Build history of the part. All positions in model axes, mm. A direction names the side the tool comes from. Round coordinates to 2 decimals unless told otherwise and drop trailing zeros. Order: outer loops, then holes, each group sorted by start corner. A loop starts at its lowest first (then second) coordinate and runs counter-clockwise, first axis right, second up. Notation, with made-up numbers: (17, 36) -> (26, 36) arc R19 ccw to (26, 53) -> close; hole circle Ø4 at (-27, 66). An arc over 180 degrees is marked (long way). Answer as CSV lines item,"result". Start each with the question number.
Autodesk Inventor part; units mm, degrees
ref_plane "YZ Plane" through (0, 0, 0) normal (1, 0, 0) x (0, 1, 0)
ref_plane "XZ Plane" through (0, 0, 0) normal (0, 1, 0) x (-1, 0, 0)
ref_plane "XY Plane" through (0, 0, 0) normal (0, 0, 1) x (1, 0, 0)
sketch "Náčrt1" plane through (0, 0, 0) normal (0, 1, 0) x (-1, 0, 0)
  line L0 (0, -68.6) -> (0, 68.6)
  line L1 (-123.9, 0) -> (123.9, 0)
  line L2 (88.5, -49) -> (-88.5, -49)
  line L3 (-88.5, -49) -> (-88.5, 49)
  line L4 (-88.5, 49) -> (88.5, 49)
  line L5 (88.5, 49) -> (88.5, -49)
  point P0 (0, 0)
  dimension "d0" = 177
  dimension "d1" = 98
extrude "Vysunutí1" add sketch "Náčrt1" along normal blind 3
sketch "Náčrt2" plane through (0, 3, 0) normal (0, 1, 0) x (1, 0, 0)
  line L0 (0, 68.6) -> (0, -68.6)
  line L1 (123.9, 0) -> (-123.9, 0)
  point P0 (0, 0)
  point P1 (-83.55, 44.05)
  point P2 (-83.55, -44.05)
  point P3 (83.55, -44.05)
  point P4 (83.55, 44.05)
  dimension "d4" = 88.1
  dimension "d5" = 167.1
  dimension "d6" = 88.1
  dimension "d7" = 167.1
hole "Díra1" at (-83.55, 3, -44.05) at (-83.55, 3, 44.05) at (83.55, 3, 44.05) at (83.55, 3, -44.05) direction (0, -1, 0) diameter 3.4 end through all
fillet "Zaoblení1" radius 3 4 edges at (88.5, 1.5, 49) (88.5, 1.5, -49) (-88.5, 1.5, 49) (-88.5, 1.5, -49)
sketch "Náčrt3" plane through (0, 3, 0) normal (0, 1, 0) x (1, 0, 0)
  line L0 (123.9, 0) -> (-123.9, 0)
  line L1 (-88.5, 46) -> (-88.5, -46)
  point P0 (0, 0)
  point P1 (-38.5, 0)
  dimension "d21" = 50
hole "Díra2" at (-38.5, 3, 0) direction (0, -1, 0) diameter 60.1 end through all
sketch "Náčrt4" plane through (0, 0, 0) normal (0, -1, 0) x (1, 0, 0)
  line L0 (0, 68.6) -> (0, -68.6)
  line L1 (-123.9, 0) -> (123.9, 0)
  point P0 (0, 0)
  point P1 (40, -15)
  dimension "d29" = 40
  dimension "d38" = 15
hole "Díra3" at (40, 0, -15) direction (0, 1, 0) diameter 47.3 end through all counterbore diameter 50.3 counterbore depth 1
sketch "Náčrt5" plane through (0, 3, 0) normal (0, 1, 0) x (1, 0, 0)
  line L0 (30.3, -22.5) -> (48.5, -22.5)
  line L1 (48.5, -22.5) -> (48.5, -34)
  line L2 (48.5, -34) -> (30.3, -34)
  line L3 (30.3, -34) -> (30.3, -22.5)
  line L4 (-85.5, -49) -> (85.5, -49)
  line L5 (88.5, -46) -> (88.5, 46)
  point P0 (0, 0)
  dimension "d39" = 18.2
  dimension "d40" = 11.5
  dimension "d41" = 15
  dimension "d43" = 40
extrude "Vysunutí2" cut sketch "Náčrt5" against normal up to surface (3 mm away)
sketch "Náčrt6" plane through (0, 3, 0) normal (0, 1, 0) x (1, 0, 0)
  line L0 (123.9, 0) -> (-123.9, 0)
  line L1 (0, 68.6) -> (0, -68.6)
  circle A0 centre (-38.5, 0) radius 30.05
  point P0 (0, 0)
  point P1 (-67.5, -29)
  point P2 (-9.5, 29)
  dimension "d46" = 29
  dimension "d49" = 29
  dimension "d57" = 29
  dimension "d58" = 29
hole "Díra4" at (-67.5, 3, 29) at (-9.5, 3, -29) direction (0, -1, 0) diameter 3.9 end through all
chamfer "Zkosení1" distance 1.5 angle 45 6 edges at (83.55, 3, -45.75) (-83.55, 3, -45.75) (83.55, 3, 42.35) (-83.55, 3, 42.35) (-9.5, 3, -30.95) (-67.5, 3, 27.05)
properties part number "4.L - GM - 01.02" material "LCP plast"
Q1. Which spindle directions (+Z, -Z, +X, -X, +Y, -Y) get a long thin tool onto all of the face, cutting with end or side? Do faces 1 (the face through (59, 1, -30)), 2 (the face through (32.9, 2.01, -37.56)). Say none if no direction does.
Q2. Slice it at C-C, the plane x = -38.5. Write the cut outline in (y, z), plus the area to 3 significant figures.
Q3. Slice it at A-A, the plane x = 40. Write the cut outline in (y, z).
Q4. Slice it at B-B, the plane z = -44.05. Write the cut outline in (x, y).
Q5. Two-plate mould, pull along X, no slides. Class faces 3 (the face through (-8.75, 0.74, -27.2)), 4 (the face through (1, 0, 1)): +X half, -X half, draft (parallel to the pull), parting line (faces both ways), or undercut.
Q6. Flat gauge pins, fed straight in: pin 1 Ø2.5 at (x, z) = (83.55, 44.05) entering from +Y; pin 2 Ø1 at (x, z) = (-69, -17.5) entering from -Y. Where does each tip first touch, or does it go through?
Q7. Probe L1, parallel to X at y = 0.95, z = -44.05; L2, parallel to Z at x = -83.55, y = 1.25; L3, parallel to Z at x = 40, y = 1.7. List the from-to ranges inside material, lowest first.
Q8. Slice it at D-D, the plane z = 12. Write the cut outline in (x, y).
Solutions:
1,face 1,"-Y"
1,face 2,"+Y, -Y"
2,outline,"(0, -49) -> (3, -49) -> (3, -30.05) -> (0, -30.05) -> close; (0, 30.05) -> (3, 30.05) -> (3, 49) -> (0, 49) -> close"
2,area,"114 mm2"
3,outline,"(0, -49) -> (3, -49) -> (3, -38.65) -> (1, -38.65) -> (1, -40.15) -> (0, -40.15) -> close; (0, 10.15) -> (1, 10.15) -> (1, 8.65) -> (3, 8.65) -> (3, 22.5) -> (0, 22.5) -> close; (0, 34) -> (3, 34) -> (3, 49) -> (0, 49) -> close"
4,outline,"(-88.5, 0) -> (-85.25, 0) -> (-85.25, 1.5) -> (-86.75, 3) -> (-88.5, 3) -> close; (-81.85, 0) -> (81.85, 0) -> (81.85, 1.5) -> (80.35, 3) -> (-80.35, 3) -> (-81.85, 1.5) -> close; (85.25, 0) -> (88.5, 0) -> (88.5, 3) -> (86.75, 3) -> (85.25, 1.5) -> close"
5,face 3,"undercut"
5,face 4,"draft"
6,pin 1,"passes through"
6,pin 2,"stops at y = 0"
7,L1,"x = -88.5 to -85.25, -81.85 to 81.85, 85.25 to 88.5"
7,L2,"z = -49 to -45.75, -42.35 to 42.35, 45.75 to 49"
7,L3,"z = -49 to -38.65, 8.65 to 22.5, 34 to 49"
8,outline,"(-88.5, 0) -> (-66.05, 0) -> (-66.05, 3) -> (-88.5, 3) -> close; (-10.95, 0) -> (88.5, 0) -> (88.5, 3) -> (-10.95, 3) -> close"
